Verification items for the finished model (mm, model axes). Face numbers are marked on the shaded views. A direction names the side the tool comes from. Give positions to 0.01 mm unless a question says otherwise; leave off trailing zeros. Write each loop counter-clockwise with the first axis right and the second up, starting at its lowest first coordinate (ties: lowest second). Pieces come first, ordered by that corner, then holes. Notation, with made-up numbers: (84.5, 75.25) -> (137.5, 75.25) arc R17 ccw to (137.5, 79.25) -> close; hole circle Ø11 at (14, 80.5). An arc over 180 degrees is marked (long way). Answer as CSV lines item,"result". Start each with the question number.
1) Sectioned sample at A-A on y = 0. Record the cut outline in (x, z) (3 decimals), and give its area (3 significant figures).
2) Gauge pin test, flat ends, axial feed: pin 1 Ø4.5 at (y, z) = (-0.5, 4.5) entering from +X; pin 2 Ø4 at (y, z) = (3, 12) entering from +X (3 decimals); pin 3 Ø8 at (y, z) = (5, 2) entering from -X; pin 4 Ø8 at (x, z) = (-1.5, 8) entering from +Y. Record the tip position at first contact, or that the pin passes through.
3) Sectioned sample at C-C on x = 2. Record the cut outline in (y, z) (3 decimals).
4) Material ranges on L1, parallel to Y at x = 3, z = 8.5; L2, parallel to Y at x = -2.5, z = 14 (3 decimals); L3, parallel to X at y = 2.75, z = 10.5, recorded low to high.
5) Tool access check on the marked faces 1, 2, 3 and 4. Record the directions out of +Z, -Z, +X, -X, +Y, -Y that give a thin tool (end or side, any length) a straight path to the whole face; none if there is none.
6) Sectioned sample at B-B on z = 7.75. Record the cut outline in (x, y) (3 decimals).
7) Sectioned sample at D-D on x = 5.5. Record the cut outline in (y, z) (3 decimals), and give its area (3 significant figures).
8) Mould release check, pull along Z, two halves, no side actions. Record for the marked faces 5, 6 and 7: released by +Z, released by -Z, zero draft, split by the parting line, or undercut.
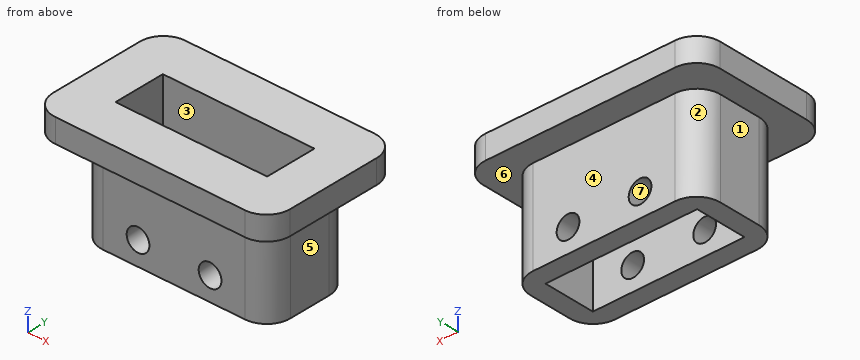
Autodesk Inventor part; units mm, degrees
ref_plane "YZ Plane" through (0, 0, 0) normal (1, 0, 0) x (0, 1, 0)
ref_plane "XZ Plane" through (0, 0, 0) normal (0, 1, 0) x (-1, 0, 0)
ref_plane "XY Plane" through (0, 0, 0) normal (0, 0, 1) x (1, 0, 0)
sketch "Sketch1" plane through (0, 0, 0) normal (0, 0, 1) x (1, 0, 0)
  line L0 (12.7, -6.0198) -> (-12.7, -6.0198)
  line L1 (-12.7, -6.0198) -> (-12.7, 6.0198)
  line L2 (-12.7, 6.0198) -> (12.7, 6.0198)
  line L3 (12.7, 6.0198) -> (12.7, -6.0198)
  line L4 (12.7, -6.0198) -> (-12.7, 6.0198) construction
  line L5 (-12.7, -6.0198) -> (12.7, 6.0198) construction
  point P0 (0, 0)
  dimension "d0" = 25.4
  dimension "d1" = 12.0396
extrude "Extrusion1" add sketch "Sketch1" along normal blind 12.7
shell "Shell1" thickness 2.54 removed faces 2 at (4.2333, -2.0066, 0) at (4.2333, -2.0066, 12.7)
sketch "Sketch2" plane through (-12.7, 6.0198, 0) normal (0, 1, 0) x (1, 0, 0)
  line L0 (-2.1226, -3.175) -> (30.0619, -3.175)
  line L1 (0, 0) -> (25.4, 0)
  circle A0 centre (7.874, -3.175) radius 1.524
  circle A1 centre (17.526, -3.175) radius 1.524
  line L2 (12.7, 1.1779) -> (12.7, -16.2415)
  point P0 (12.7, 0)
  point P1 (12.7, 0)
  dimension "d23" = 3.175
  dimension "d24" = 3.048
  dimension "d25" = 9.652
extrude "Extrusion2" cut sketch "Sketch2" against normal through all
sketch "Sketch3" plane through (0, 0, 12.7) normal (0, 0, 1) x (1, 0, 0)
  line L0 (-10.16, 3.4798) -> (10.16, 3.4798)
  line L1 (10.16, 3.4798) -> (10.16, -3.4798)
  line L2 (10.16, -3.4798) -> (-10.16, -3.4798)
  line L3 (-10.16, -3.4798) -> (-10.16, 3.4798)
  line L4 (-10.16, 3.4798) -> (10.16, -3.4798) construction
  line L5 (10.16, 3.4798) -> (-10.16, -3.4798) construction
  line L6 (-12.7, 9.525) -> (12.7, 9.525)
  line L7 (15.875, 6.35) -> (15.875, -6.35)
  line L8 (12.7, -9.525) -> (-12.7, -9.525)
  line L9 (-15.875, -6.35) -> (-15.875, 6.35)
  line L10 (-15.875, 9.525) -> (15.875, -9.525) construction
  line L11 (15.875, 9.525) -> (-15.875, -9.525) construction
  arc A0 (12.7, -9.525) -> (15.875, -6.35) centre (12.7, -6.35) ccw
  arc A1 (15.875, 6.35) -> (12.7, 9.525) centre (12.7, 6.35) ccw
  arc A2 (-12.7, 9.525) -> (-15.875, 6.35) centre (-12.7, 6.35) ccw
  arc A3 (-15.875, -6.35) -> (-12.7, -9.525) centre (-12.7, -6.35) ccw
  point P0 (0, 0)
  dimension "d28" = 19.05
  dimension "d29" = 31.75
  dimension "d30" = 3.175
extrude "Extrusion3" add sketch "Sketch3" along normal blind 3.175
fillet "Fillet1" radius 3.175 4 edges at (12.7, 6.0198, 6.35) (12.7, -6.0198, 6.35) (-12.7, 6.0198, 6.35) (-12.7, -6.0198, 6.35)
properties part number "E-Stop_Fixture"
Ans:
1,outline,"(-15.875, 12.7) -> (-12.7, 12.7) -> (-12.7, 0) -> (-10.16, 0) -> (-10.16, 15.875) -> (-15.875, 15.875) -> close; (10.16, 0) -> (12.7, 0) -> (12.7, 12.7) -> (15.875, 12.7) -> (15.875, 15.875) -> (10.16, 15.875) -> close"
1,area,"101 mm²"
2,pin 1,"stops at x = 12.7"
2,pin 2,"stops at x = 15.875"
2,pin 3,"stops at x = -12.7"
2,pin 4,"stops at y = 6.02"
3,outline,"(-9.525, 12.7) -> (-6.02, 12.7) -> (-6.02, 0) -> (-3.48, 0) -> (-3.48, 15.875) -> (-9.525, 15.875) -> close; (3.48, 0) -> (6.02, 0) -> (6.02, 12.7) -> (9.525, 12.7) -> (9.525, 15.875) -> (3.48, 15.875) -> close"
4,L1,"y = -6.02 to -3.48, 3.48 to 6.02"
4,L2,"y = -9.525 to -3.48, 3.48 to 9.525"
4,L3,"x = -12.7 to -10.16, 10.16 to 12.7"
5,face 1,"-Z, -X, +Y, -Y"
5,face 2,"-Z, -X, +Y"
5,face 3,"+Z, -Z"
5,face 4,"-Z, +X, -X, +Y"
6,outline,"(-12.7, -2.845) arc R3.175 ccw to (-9.525, -6.02) -> (9.525, -6.02) arc R3.175 ccw to (12.7, -2.845) -> (12.7, 2.845) arc R3.175 ccw to (9.525, 6.02) -> (-9.525, 6.02) arc R3.175 ccw to (-12.7, 2.845) -> close; hole (-10.16, -3.48) -> (10.16, -3.48) -> (10.16, 3.48) -> (-10.16, 3.48) -> close"
7,outline,"(-9.525, 12.7) -> (-6.02, 12.7) -> (-6.02, 4.542) -> (-3.48, 4.542) -> (-3.48, 15.875) -> (-9.525, 15.875) -> close; (-6.02, 0) -> (-3.48, 0) -> (-3.48, 1.808) -> (-6.02, 1.808) -> close; (3.48, 0) -> (6.02, 0) -> (6.02, 1.808) -> (3.48, 1.808) -> close; (3.48, 4.542) -> (6.02, 4.542) -> (6.02, 12.7) -> (9.525, 12.7) -> (9.525, 15.875) -> (3.48, 15.875) -> close"
7,area,"89.0 mm²"
8,face 5,"zero draft"
8,face 6,"released by -Z"
8,face 7,"undercut"
